```python
from build123d import *

# Parameters (mm, degrees)
SKETCH4_W                        = 53.34
SKETCH4_H                        = 53.34
BOSS_EXTRUDE2_DEPTH              = 25.4
SHELL1_T                         = -1.27
SKETCH13_W                       = 14.8000212
SKETCH13_H                       = 5.334
SKETCH13_W_2                     = 8.999982
SKETCH13_H_2                     = 12.7
CUT_EXTRUDE5_DEPTH               = 1.27
F_1_2_CLEARANCE_HOLE2_D          = 13.49248
F_1_2_CLEARANCE_HOLE2_DEPTH      = 1.27
F_97_0_0059_DIAMETER_HOLE1_D     = 7.62
F_97_0_0059_DIAMETER_HOLE1_DEPTH = 1.27
FILLET2_R                        = 1.27
CUT_EXTRUDE6_REACH               = 55.34
SKETCH24_W                       = 31.75
SKETCH24_H                       = 6.35
CUT_EXTRUDE7_REACH               = 55.34
SKETCH26_W                       = 26.67
SKETCH26_H                       = 6.35
SKETCH27_R                       = 1.4732
BOSS_EXTRUDE3_DEPTH              = 24.13
SKETCH28_R                       = 1.4732
CUT_EXTRUDE8_DEPTH               = 26.4
BODY_MOVE_COPY1_ANGLE            = 180


with BuildPart() as part:
    # Sketch4 → Boss-Extrude2 (new body)
    with BuildSketch(Plane(origin=(0, 0, 0), x_dir=(1, 0, 0), z_dir=(0, 1, 0))):
        with Locations((25.4, 25.4)):
            Rectangle(SKETCH4_W, SKETCH4_H)
    extrude(amount=BOSS_EXTRUDE2_DEPTH)

    # Shell1
    shell1_openings = [part.faces().sort_by_distance(p)[0] for p in [
        (25.4, 0, -25.4),
    ]]
    offset(amount=SHELL1_T, openings=shell1_openings, kind=Kind.INTERSECTION)

    # Sketch13 → Cut-Extrude5 (cut)
    with BuildSketch(Plane(origin=(0, 0, -52.07), x_dir=(-1, 0, 0), z_dir=(0, 0, -1))):
        with Locations((-39.37, 2.667)):
            Rectangle(SKETCH13_W, SKETCH13_H)
        with Locations((-8.89, 6.35)):
            Rectangle(SKETCH13_W_2, SKETCH13_H_2)
    extrude(amount=-CUT_EXTRUDE5_DEPTH, mode=Mode.SUBTRACT)

    # 1/2 Clearance Hole2
    with Locations(Plane.XY.offset(1.27)):
        with Locations((11.43, 15.875), (39.37, 15.875)):
            Hole(F_1_2_CLEARANCE_HOLE2_D / 2, depth=F_1_2_CLEARANCE_HOLE2_DEPTH)

    # #97 (0.0059) Diameter Hole1
    with Locations(Plane.XY.offset(1.27)):
        with Locations((24.13, 15.875)):
            Hole(F_97_0_0059_DIAMETER_HOLE1_D / 2, depth=F_97_0_0059_DIAMETER_HOLE1_DEPTH)

    # Fillet2
    fillet2_edges = [part.edges().sort_by_distance(p)[0] for p in [
        (52.07, 25.4, -25.4),
        (25.4, 25.4, -52.07),
        (-1.27, 25.4, -25.4),
        (25.4, 25.4, 1.27),
        (-1.27, 12.7, -52.07),
        (52.07, 12.7, -52.07),
        (52.07, 12.7, 1.27),
        (-1.27, 12.7, 1.27),
    ]]
    fillet(fillet2_edges, radius=FILLET2_R)

    # Sketch24 → Cut-Extrude6 (cut, up to next)
    with BuildSketch(Plane(origin=(52.07, 0, 0), x_dir=(0, 0, -1), z_dir=(1, 0, 0)), mode=Mode.PRIVATE) as cut_extrude6_sk1:
        with Locations((19.685, 3.175)):
            Rectangle(SKETCH24_W, SKETCH24_H)
    cut_extrude6_tool1 = extrude(cut_extrude6_sk1.sketch, amount=-CUT_EXTRUDE6_REACH, mode=Mode.PRIVATE) & part.part
    add(cut_extrude6_tool1.solids().sort_by_distance((52.07, 3.175, -19.685))[0], mode=Mode.SUBTRACT)

    # Sketch26 → Cut-Extrude7 (cut, up to next)
    with BuildSketch(Plane.ZY.offset(1.27), mode=Mode.PRIVATE) as cut_extrude7_sk1:
        with Locations((-17.145, 3.175)):
            Rectangle(SKETCH26_W, SKETCH26_H)
    cut_extrude7_tool1 = extrude(cut_extrude7_sk1.sketch, amount=-CUT_EXTRUDE7_REACH, mode=Mode.PRIVATE) & part.part
    add(cut_extrude7_tool1.solids().sort_by_distance((-1.27, 3.175, -17.145))[0], mode=Mode.SUBTRACT)

    # Sketch27 → Boss-Extrude3 (add)
    with BuildSketch(Plane.XZ.offset(-24.13)):
        with BuildLine():
            Line((1.905, -3.7592), (0, -3.7592))
            Line((0, -3.7592), (0, 0))
            Line((0, 0), (3.7592, 0))
            Line((3.7592, 0), (3.7592, -1.905))
            ThreePointArc((3.7592, -1.905), (3.216117394, -3.216117394), (1.905, -3.7592))
        make_face()
        with Locations((1.905, -1.905)):
            Circle(SKETCH27_R, mode=Mode.SUBTRACT)
        with BuildLine():
            Line((0, -47.0408), (0, -50.8))
            Line((0, -50.8), (3.7592, -50.8))
            Line((3.7592, -50.8), (3.7592, -48.895))
            ThreePointArc((3.7592, -48.895), (3.216117394, -47.583882606), (1.905, -47.0408))
            Line((1.905, -47.0408), (0, -47.0408))
        make_face()
        with Locations((1.905, -48.895)):
            Circle(SKETCH27_R, mode=Mode.SUBTRACT)
        with BuildLine():
            Line((50.8, -50.8), (47.0408, -50.8))
            Line((47.0408, -50.8), (47.0408, -48.895))
            ThreePointArc((47.0408, -48.895), (47.583882606, -47.583882606), (48.895, -47.0408))
            Line((48.895, -47.0408), (50.8, -47.0408))
            Line((50.8, -47.0408), (50.8, -50.8))
        make_face()
        with Locations((48.895, -48.895)):
            Circle(SKETCH27_R, mode=Mode.SUBTRACT)
        with BuildLine():
            Line((47.0408, 0), (47.0408, -1.905))
            ThreePointArc((47.0408, -1.905), (47.583882606, -3.216117394), (48.895, -3.7592))
            Line((48.895, -3.7592), (50.8, -3.7592))
            Line((50.8, -3.7592), (50.8, 0))
            Line((50.8, 0), (47.0408, 0))
        make_face()
        with Locations((48.895, -1.905)):
            Circle(SKETCH27_R, mode=Mode.SUBTRACT)
    extrude(amount=BOSS_EXTRUDE3_DEPTH)

    # Sketch28 → Cut-Extrude8 (cut, through all)
    with BuildSketch(Plane.XZ):
        with Locations((48.895, -1.905)):
            Circle(SKETCH28_R)
        with Locations((1.905, -1.905)):
            Circle(SKETCH28_R)
        with Locations((1.905, -48.895)):
            Circle(SKETCH28_R)
        with Locations((48.895, -48.895)):
            Circle(SKETCH28_R)
    extrude(amount=-CUT_EXTRUDE8_DEPTH, mode=Mode.SUBTRACT)


with BuildPart() as part_1:
    # Body-Move/Copy1: moved
    add(part.part.rotate(Axis((25.4, 12.7, 0), (0, 0, 1)), BODY_MOVE_COPY1_ANGLE))


solid = part_1.part
```
Build history of the part. All positions in model axes, mm. A direction names the side the tool comes from. Round coordinates to 2 decimals unless told otherwise and drop trailing zeros. Loops run counter-clockwise (first coordinate to the right, second up) from the corner with the lowest first, then second, coordinate; pieces in that order, holes last.
Item 1: Saw through at C-C (z = -44). List the corners of the cut face in (x, y), then the cut area to 3 significant figures.
Item 2: Pin check, flat tips, straight feed: P1, Ø4, axis at x = 33.5, z = -11, coming from the +Y side; P2, Ø11, axis at x = 11.43, y = 9.525, coming from the +Z side. Stop position of each tip, or through.
Item 3: Saw through at A-A (x = 39.37). List the corners of the cut face in (y, z), then the cut area to 3 significant figures.
Item 4: Two-plate mould, pull along X, no slides. Class faces 1 (the face through (50, 13, -47.041)), 2 (the face through (18.83, 23, -51)), 3 (the face through (52.07, 14, -25)), 4 (the face through (-1.27, 14, -25)): released by +X, released by -X, zero draft, split by the parting line, or undercut.
Item 5: Saw through at B-B (y = 17.75). State how many separate pieces and enclosed holes the cut face has, then the cut area to 3 significant figures.
Item 6: Drill centre lines: line 1 along X through (y, z) = (4.25, -2); line 2 along Z through (x, y) = (13, 19.25); line 3 along X through (y, z) = (6.5, -29). Where is each one in solid material? Low to high.
Item 7: Which spindle directions (+Z, -Z, +X, -X, +Y, -Y) get a long thin tool onto all of the face, cutting with end or side? Do faces 5 (the face through (-1, 22, -35.56)), 6 (the face through (-0.888, 13.166, -51.708)), 7 (the face through (50, 13, -3.759)), 8 (the face through (-1, 22, -3.81)), 9 (the face through (28, 25.4, -51)). Say none if no direction does.
Worked answers:
1. outline: (-1.27, 1.27) arc R1.27 ccw to (0, 0) - (50.8, 0) arc R1.27 ccw to (52.07, 1.27) - (52.07, 25.4) - (50.8, 25.4) - (50.8, 1.27) - (0, 1.27) - (0, 25.4) - (-1.27, 25.4) - close
1. area: 128 mm2
2. P1: stops at y = 1.27
2. P2: stops at z = -50.8
3. outline: (0, -50.8) arc R1.27 ccw to (1.27, -52.07) - (12.7, -52.07) - (12.7, -50.8) - (1.27, -50.8) - (1.27, 0) - (2.78, 0) - (2.78, 1.27) - (1.27, 1.27) arc R1.27 ccw to (0, 0) - close; (16.27, 0) - (25.4, 0) - (25.4, 1.27) - (16.27, 1.27) - close
3. area: 95.1 mm2
4. face 1: undercut
4. face 2: undercut
4. face 3: released by +X
4. face 4: released by -X
5. separate pieces: 1
5. enclosed holes: 4
5. area: 278 mm2
6. line 1: x = -1.27 to 0.43, 3.38 to 3.76, 47.04 to 47.42, 50.37 to 52.07
6. line 2: z = -52.07 to -50.8, 0 to 1.27
6. line 3: x = -1.27 to 0, 50.8 to 52.07
7. face 5: -X, +Y
7. face 6: -Z, -X, +Y, -Y
7. face 7: +Y
7. face 8: +X, -X, +Y
7. face 9: +Z, -Z, +X, -X, +Y
